The listing builds one solid part. Answer for the finished solid, in the listing's coordinates (mm). Face numbers are marked on the shaded views. Coordinates: 2 decimals unless noted, no trailing zeros. Order: outer loops, then holes, each group sorted by start corner. A loop starts at its lowest first (then second) coordinate and runs counter-clockwise, first axis right, second up. Notation, with made-up numbers: (88.5, 82) -> (143.5, 82) arc R12 cw to (143.5, 101) -> close; hole circle Ø5 at (-38.75, -28.75). An arc over 180 degrees is marked (long way). Answer in a Markdown table with one row per item. Add a question column.
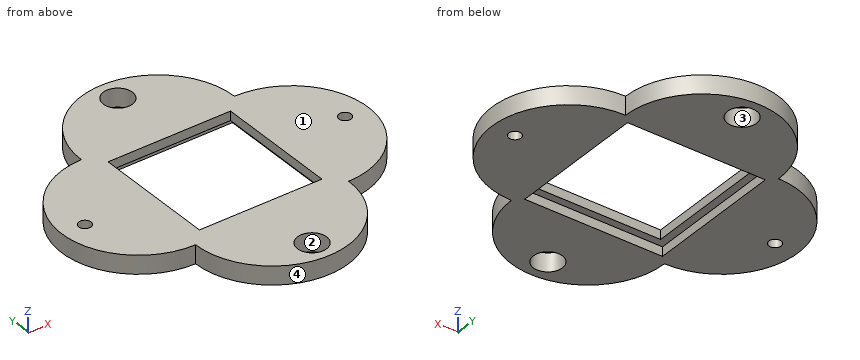
```python
from build123d import *

# Parameters (mm, degrees)
IZIM1_R                     = 9.5
IZIM1_R_2                   = 4
IZIM1_W                     = 90
IZIM1_H                     = 90
Y_KSEKLIK_EKSTR_ZYON1_DEPTH = 12
IZIM2_W                     = 90
IZIM2_H                     = 90
IZIM2_W_2                   = 80
IZIM2_H_2                   = 80
Y_KSEKLIK_EKSTR_ZYON2_DEPTH = 6


with BuildPart() as part:
    # Çizim1 → Yükseklik-Ekstrüzyon1 (new body)
    with BuildSketch(Plane.XY):
        with BuildLine():
            ThreePointArc((45.945945946, 48.048048048), (-4.054054054, 98.048048048), (-54.054054054, 48.048048048))
            ThreePointArc((-54.054054054, 48.048048048), (-104.054054054, -1.951951952), (-54.054054054, -51.951951952))
            ThreePointArc((-54.054054054, -51.951951952), (-4.054054054, -101.951951952), (45.945945946, -51.951951952))
            ThreePointArc((45.945945946, -51.951951952), (95.945945946, -1.951951952), (45.945945946, 48.048048048))
        make_face()
        with Locations((-4.054054054, -86.951951952)):
            Circle(IZIM1_R, mode=Mode.SUBTRACT)
        with Locations((-89.054054054, -1.951951952)):
            Circle(IZIM1_R_2, mode=Mode.SUBTRACT)
        with Locations((-4.054054054, 83.048048048)):
            Circle(IZIM1_R, mode=Mode.SUBTRACT)
        with Locations((80.945945946, -1.951951952)):
            Circle(IZIM1_R_2, mode=Mode.SUBTRACT)
        with Locations((-4.054054054, -1.951951952)):
            Rectangle(IZIM1_W, IZIM1_H, mode=Mode.SUBTRACT)
    extrude(amount=Y_KSEKLIK_EKSTR_ZYON1_DEPTH)

    # Çizim2 → Yükseklik-Ekstrüzyon2 (add)
    with BuildSketch(Plane.XY.offset(12)):
        with Locations((-4.054054054, -1.951951952)):
            Rectangle(IZIM2_W, IZIM2_H)
        with Locations((-4.054054054, -1.951951952)):
            Rectangle(IZIM2_W_2, IZIM2_H_2, mode=Mode.SUBTRACT)
    extrude(amount=-Y_KSEKLIK_EKSTR_ZYON2_DEPTH)


solid = part.part
```
Q1. Given pin 1 (5 mm diameter, centred on y = -65.5, z = 1.5, fed in from +X); pin 2 (4 mm diameter, centred on y = -12, z = 1.5, fed in from -X); pin 3 (3 mm diameter, centred on y = 3.5, z = 10, fed in from -X); pin 4 (11.5 mm diameter, centred on x = -4.05, y = 83.05, fed in from +Z), each flat-ended and moving along its own axis, determine where each tip first touches the part or whether it passes through.
Q2. A cutting plane is placed at A-A (y = -81). Determine the outline of the cut face in (x, z).
Q3. A cutting plane is placed at B-B (x = 25). Determine the outline of the cut face in (y, z), then the cut area to 3 significant figures.
Q4. Determine the mould class of the marked faces 1, 2, 3 and 4 for opening direction X: +X half, -X half, draft (parallel to the pull), parting line (faces both ways), or undercut.
Q5. A cutting plane is placed at C-C (z = 9.5). Determine the outline of the cut face in (x, y).
Q6. A cutting plane is placed at D-D (y = 14). Determine the outline of the cut face in (x, z), then the cut area to 3 significant figures.
Q7. Straight lines are drawn through the part: line 1 (Y direction, x = -1.5, z = 1.5); line 2 (Y direction, x = -1, z = 0.75); line 3 (Y direction, x = -30.5, z = 8). For each, find the intervals that lie inside material, in ascending order.
Returned:
| question | item | result |
|---|---|---|
| 1 | pin 1 | stops at x = 44.71 |
| 1 | pin 2 | stops at x = -103.4 |
| 1 | pin 3 | stops at x = -103.9 |
| 1 | pin 4 | passes through |
| 2 | outline | (-44.75, 0) -> (-11.46, 0) -> (-11.46, 12) -> (-44.75, 12) -> close; (3.35, 0) -> (36.64, 0) -> (36.64, 12) -> (3.35, 12) -> close |
| 3 | outline | (-92.64, 0) -> (-46.95, 0) -> (-46.95, 6) -> (-41.95, 6) -> (-41.95, 12) -> (-92.64, 12) -> close; (38.05, 6) -> (43.05, 6) -> (43.05, 0) -> (88.74, 0) -> (88.74, 12) -> (38.05, 12) -> close |
| 3 | area | 1,160 mm² |
| 4 | face 1 | draft |
| 4 | face 2 | undercut |
| 4 | face 3 | undercut |
| 4 | face 4 | parting line |
| 5 | outline | (-54.05, -51.95) arc R50 ccw to (45.95, -51.95) arc R50 ccw to (45.95, 48.05) arc R50 ccw to (-54.05, 48.05) arc R50 ccw to start; hole circle Ø8 at (-89.05, -1.95); hole (-44.05, -41.95) -> (35.95, -41.95) -> (35.95, 38.05) -> (-44.05, 38.05) -> close; hole circle Ø19 at (-4.05, -86.95); hole circle Ø19 at (-4.05, 83.05); hole circle Ø8 at (80.95, -1.95) |
| 6 | outline | (-101.44, 0) -> (-49.05, 0) -> (-49.05, 6) -> (-44.05, 6) -> (-44.05, 12) -> (-101.44, 12) -> close; (35.95, 6) -> (40.95, 6) -> (40.95, 0) -> (93.33, 0) -> (93.33, 12) -> (35.95, 12) -> close |
| 6 | area | 1,320 mm² |
| 7 | line 1 | y = -101.89 to -96.1, -77.8 to -46.95, 43.05 to 73.9, 92.2 to 97.98 |
| 7 | line 2 | y = -101.86 to -95.95, -77.96 to -46.95, 43.05 to 74.05, 92.04 to 97.95 |
| 7 | line 3 | y = -94.39 to -41.95, 38.05 to 90.48 |
